from build123d import *

# Parameters (mm, degrees)
SKETCH1_R           = 23
SKETCH1_R_2         = 18
BOSS_EXTRUDE1_DEPTH = 7
BOSS_EXTRUDE2_DEPTH = 7
CUT_EXTRUDE1_DEPTH  = 7
BOSS_EXTRUDE3_DEPTH = 7
SKETCH7_R           = 2.2
CUT_EXTRUDE2_DEPTH  = 7
CUT_EXTRUDE3_DEPTH  = 7


with BuildPart() as part:
    # Sketch1 → Boss-Extrude1 (new body)
    with BuildSketch(Plane.XY):
        Circle(SKETCH1_R)
        Circle(SKETCH1_R_2, mode=Mode.SUBTRACT)
    extrude(amount=BOSS_EXTRUDE1_DEPTH)

    # Sketch3 → Boss-Extrude2 (add)
    with BuildSketch(Plane.XY):
        with BuildLine():
            Line((-23.80139919, -18.167885182), (-0.617388595, -29.936557696))
            Line((-0.617388595, -29.936557696), (3.003741409, -22.803015975))
            ThreePointArc((3.003741409, -22.803015975), (-10.410748762, -20.508932449), (-20.180269185, -11.034343461))
            Line((-20.180269185, -11.034343461), (-23.80139919, -18.167885182))
        make_face()
    extrude(amount=BOSS_EXTRUDE2_DEPTH)

    # Sketch5 → Cut-Extrude1 (cut)
    with BuildSketch(Plane.XY):
        with BuildLine():
            Line((-15.062285021, -9.855332057), (-17.325491273, -14.313795633))
            Line((-17.325491273, -14.313795633), (-1.328523963, -22.434179668))
            Line((-1.328523963, -22.434179668), (0.93468229, -17.975716092))
            ThreePointArc((0.93468229, -17.975716092), (-8.14754251, -16.050468873), (-15.062285021, -9.855332057))
        make_face()
    extrude(amount=CUT_EXTRUDE1_DEPTH, mode=Mode.SUBTRACT)

    # Sketch6 → Boss-Extrude3 (add)
    with BuildSketch(Plane.XY):
        with BuildLine():
            ThreePointArc((-22.555487137, -4.5), (-26.136916399, 0), (-22.555487137, 4.5))
            ThreePointArc((-22.555487137, 4.5), (-23, 0), (-22.555487137, -4.5))
        make_face()
        with BuildLine():
            ThreePointArc((22.555487137, -4.5), (25.860234666, 0), (22.555487137, 4.5))
            ThreePointArc((22.555487137, 4.5), (23, 0), (22.555487137, -4.5))
        make_face()
    extrude(amount=BOSS_EXTRUDE3_DEPTH)

    # Sketch7 → Cut-Extrude2 (cut)
    with BuildSketch(Plane.XY):
        with Locations((-21.5, 0)):
            Circle(SKETCH7_R)
        with Locations((21.5, 0)):
            Circle(SKETCH7_R)
    extrude(amount=CUT_EXTRUDE2_DEPTH, mode=Mode.SUBTRACT)

    # Sketch8 → Cut-Extrude3 (cut)
    with BuildSketch(Plane.XY):
        Polygon((-14.382905313, -15.80751176), (-4.271109923, -20.940463541), (-5.629033675, -23.615541687), (-15.740829065, -18.482589905), align=None)
    extrude(amount=CUT_EXTRUDE3_DEPTH, mode=Mode.SUBTRACT)


solid = part.part
The listing builds one solid part. Answer for the finished solid, in the listing's coordinates (mm). A direction names the side the tool comes from. Give positions to 0.01 mm unless a question says otherwise; leave off trailing zeros. Write each loop counter-clockwise with the first axis right and the second up, starting at its lowest first coordinate (ties: lowest second). Pieces come first, ordered by that corner, then holes.
1) Section B-B (z = 3.75) is taken. Write down the section's boundary in (x, y).
2) For a pull along Y with two mould halves and no side action, classify faces 1 (the face through (-12.37, -23.97, 3.45)), 2 (the face through (-2.82, -21.677, 3.451)), 3 (the face through (0, 23, 3)), 4 (the face through (-21.633, -7.812, 3.451)) as pulls with the +Y half, pulls with the -Y half, needs draft (parallel to the pull), parting line crosses it, or undercut.
3) Section D-D (x = -21.5) is taken. Write down the section's boundary in (y, z), and give its area (3 significant figures).
4) Section A-A (y = 0) is taken. Write down the section's boundary in (x, z).
5) Section C-C (x = 4) is taken. Write down the section's boundary in (y, z), and give its area (3 significant figures).
6) Given P1, Ø12, axis at x = 1.5, y = -7, coming from the +Z side; P2, Ø3, axis at y = 9, z = 1.5, coming from the -X side; P3, Ø1.5, axis at y = 3, z = 2.5, coming from the -X side, each flat-ended and moving along its own axis, determine where each tip first touches the part or whether it passes through.
7) A tool of negligible diameter and unlimited length cuts with its end or side. For faces 5 (the face through (-21.965, -14.551, 3.451)), 6 (the face through (25.86, -0.08, 3.45)), 7 (the face through (-15.875, -15.05, 3.451)), from which of +Z, -Z, +X, -X, +Y, -Y can it reach the whole face along a straight path? Write none if from no direction.
8) Find the intervals of material crossed by L1, parallel to X at y = 16, z = 1.25; L2, parallel to X at y = -4, z = 0.5; L3, parallel to Y at x = 15, z = 3.5, in increasing order.
Response:
1. outline: (-23.8, -18.17) - (-0.62, -29.94) - (3, -22.8) arc R23 ccw to (22.56, -4.5) arc R4.72 ccw to (22.56, 4.5) arc R23 ccw to (-22.56, 4.5) arc R4.62 ccw to (-22.56, -4.5) arc R23 ccw to (-20.18, -11.03) - close; hole circle Ø4.4 at (-21.5, 0); hole (-17.33, -14.31) - (-14.38, -15.81) - (-15.74, -18.48) - (-5.63, -23.62) - (-4.27, -20.94) - (-1.33, -22.43) - (0.93, -17.98) arc R18 ccw (long way) to (-15.06, -9.86) - close; hole circle Ø4.4 at (21.5, 0)
2. face 1: pulls with the -Y half
2. face 2: undercut
2. face 3: pulls with the +Y half
2. face 4: undercut
3. outline: (-19.34, 0) - (-13.63, 0) - (-13.63, 7) - (-19.34, 7) - close; (-8.17, 0) - (-2.2, 0) - (-2.2, 7) - (-8.17, 7) - close; (2.2, 0) - (8.17, 0) - (8.17, 7) - (2.2, 7) - close
3. area: 123 mm2
4. outline: (-26.14, 0) - (-23.7, 0) - (-23.7, 7) - (-26.14, 7) - close; (-19.3, 0) - (-18, 0) - (-18, 7) - (-19.3, 7) - close; (18, 0) - (19.3, 0) - (19.3, 7) - (18, 7) - close; (23.7, 0) - (25.86, 0) - (25.86, 7) - (23.7, 7) - close
5. outline: (-22.65, 0) - (-17.55, 0) - (-17.55, 7) - (-22.65, 7) - close; (17.55, 0) - (22.65, 0) - (22.65, 7) - (17.55, 7) - close
5. area: 71.4 mm2
6. P1: passes through
6. P2: stops at x = -21.74
6. P3: stops at x = -25.55
7. face 5: +Z, -Z, -X
7. face 6: +Z, -Z, +X
7. face 7: +Z, -Z
8. L1: x = -16.52 to -8.25, 8.25 to 16.52
8. L2: x = -23.83 to -17.55, 17.55 to 23.64
8. L3: y = -17.44 to -9.95, 9.95 to 17.44
